from build123d import *

# Parameters (mm, degrees)
SKETCH1_W           = 53.34
SKETCH1_H           = 25.4
BOSS_EXTRUDE1_DEPTH = 53.34
FILLET1_R           = 5.08
SKETCH2_W           = 40.64
SKETCH2_H           = 40.64
CUT_EXTRUDE1_DEPTH  = 17.78
FILLET2_R           = 5.08


with BuildPart() as part:
    # Sketch1 → Boss-Extrude1 (new body)
    with BuildSketch(Plane(origin=(0, 0, 0), x_dir=(1, 0, 0), z_dir=(0, 1, 0))):
        with Locations((26.67, 12.7)):
            Rectangle(SKETCH1_W, SKETCH1_H)
    extrude(amount=BOSS_EXTRUDE1_DEPTH)

    # Fillet1
    fillet1_edges = [part.edges().sort_by_distance(p)[0] for p in [
        (53.34, 53.34, -12.7),
        (0, 53.34, -12.7),
        (53.34, 0, -12.7),
        (0, 0, -12.7),
    ]]
    fillet(fillet1_edges, radius=FILLET1_R)

    # Sketch2 → Cut-Extrude1 (cut)
    with BuildSketch(Plane(origin=(0, 0, -25.4), x_dir=(-1, 0, 0), z_dir=(0, 0, -1))):
        with Locations((-26.67, 26.67)):
            Rectangle(SKETCH2_W, SKETCH2_H)
    extrude(amount=-CUT_EXTRUDE1_DEPTH, mode=Mode.SUBTRACT)

    # Fillet2
    fillet2_edges = [part.edges().sort_by_distance(p)[0] for p in [
        (46.99, 6.35, -16.51),
        (46.99, 46.99, -16.51),
        (6.35, 46.99, -16.51),
        (6.35, 6.35, -16.51),
    ]]
    fillet(fillet2_edges, radius=FILLET2_R)


solid = part.part
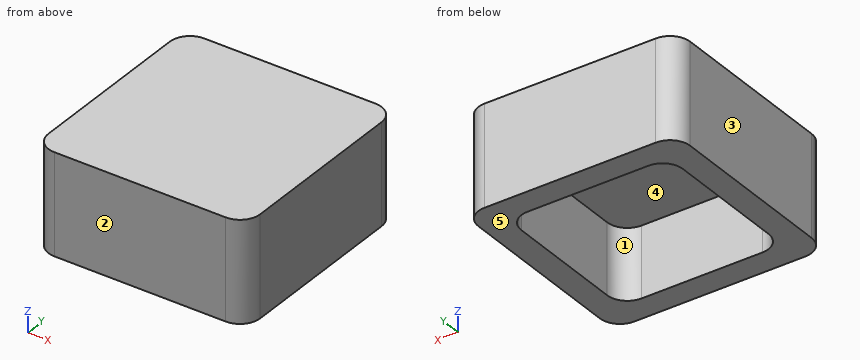
Check sheet for the modelled part. Datum: model origin and axes. Units: mm. Face numbers are marked on the shaded views. A direction names the side the tool comes from. Round coordinates to 2 decimals unless told otherwise and drop trailing zeros. Order: outer loops, then holes, each group sorted by start corner. A loop starts at its lowest first (then second) coordinate and runs counter-clockwise, first axis right, second up. Notation, with made-up numbers: M 64,64 L 114,64 A37 ccw 114,102 Z; hole C 83.25,16 d1. An arc over 180 degrees is marked long. One line per item, written item: value. Start each with the question number.
1. Scan lines: line 1 along X through (y, z) = (30.5, -9.5); line 2 along Z through (x, y) = (24, 17). Record each from-to range of solid material in increasing order.
2. Gauge pin test, flat end, axial feed: P1, Ø3, axis at x = 29, y = 10, coming from the -Z side. Record the tip position at first contact, or that the pin passes through.
3. Release check for a two-part mould opening along X. For the marked faces 3, 4 and 5 record: released by +X, released by -X, zero draft, split by the parting line, or undercut.
4. Access from +Z, -Z, +X, -X, +Y, -Y to the whole of each face (thin tool, end or side, straight path). Record for the marked faces 1 and 2.
5. Section check A-A on z = -17.25. Enter the section's corners in (x, y).
6. Section check B-B on x = 33.5. Enter the section's corners in (y, z), and give its area (3 significant figures).
Results found:
1. line 1: 0 to 6.35, 46.99 to 53.34
1. line 2: -7.62 to 0
2. P1: z = -7.62
3. face 3: released by -X
3. face 4: undercut
3. face 5: zero draft
4. face 1: -Z
4. face 2: +Z, -Z, +X, -X, -Y
5. outline: M 0,5.08 A5.08 ccw 5.08,0 L 48.26,0 A5.08 ccw 53.34,5.08 L 53.34,48.26 A5.08 ccw 48.26,53.34 L 5.08,53.34 A5.08 ccw 0,48.26 Z; hole M 6.35,11.43 A5.08 ccw 11.43,6.35 L 41.91,6.35 A5.08 ccw 46.99,11.43 L 46.99,41.91 A5.08 ccw 41.91,46.99 L 11.43,46.99 A5.08 ccw 6.35,41.91 Z
6. outline: M 0,-25.4 L 6.35,-25.4 L 6.35,-7.62 L 46.99,-7.62 L 46.99,-25.4 L 53.34,-25.4 L 53.34,0 L 0,0 Z
6. area: 632 mm^2
